Read the model definition and answer for the solid it produces. Units are mm, in the model's axes. Face numbers are marked on the shaded views. A direction names the side the tool comes from. Round coordinates to 2 decimals unless told otherwise and drop trailing zeros. Order: outer loops, then holes, each group sorted by start corner. A loop starts at its lowest first (then second) coordinate and runs counter-clockwise, first axis right, second up.
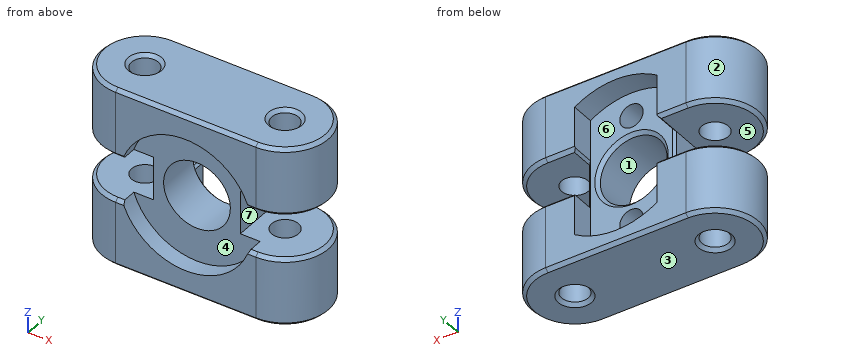
from build123d import *

# Parameters (mm, degrees)
SKETCH1_W           = 21
SKETCH1_H           = 27
BOSS_EXTRUDE1_DEPTH = 13
SKETCH8_R           = 6.5
BOSS_EXTRUDE2_DEPTH = 27
SKETCH2_R           = 5
CUT_EXTRUDE1_DEPTH  = 13
SKETCH3_W           = 21.50173114
SKETCH3_H           = 6.5
CUT_EXTRUDE2_DEPTH  = 13
SKETCH7_W           = 13
SKETCH7_H           = 6.5
CUT_EXTRUDE7_DEPTH  = 3.5
SKETCH4_R           = 2
CUT_EXTRUDE3_DEPTH  = 35
CUT_EXTRUDE4_DEPTH  = 3.5
SKETCH6_R           = 1.75
CUT_EXTRUDE5_DEPTH  = 6
CHAMFER1_SIZE       = 0.5
CHAMFER2_SIZE       = 0.35
CHAMFER3_SIZE       = 0.35
SKETCH9_R           = 10
CUT_EXTRUDE8_DEPTH  = 2.5


with BuildPart() as part:
    # Sketch1 → Boss-Extrude1 (new body)
    with BuildSketch(Plane(origin=(0, 0, 0), x_dir=(1, 0, 0), z_dir=(0, 1, 0))):
        Rectangle(SKETCH1_W, SKETCH1_H)
    extrude(amount=BOSS_EXTRUDE1_DEPTH)

    # Sketch8 → Boss-Extrude2 (add)
    with BuildSketch(Plane(origin=(0, 0, -13.5), x_dir=(-1, 0, 0), z_dir=(0, 0, -1))):
        with Locations((-10.5, 6.5)):
            Circle(SKETCH8_R)
        with Locations((10.5, 6.5)):
            Circle(SKETCH8_R)
    extrude(amount=-BOSS_EXTRUDE2_DEPTH)

    # Sketch2 → Cut-Extrude1 (cut)
    with BuildSketch(Plane(origin=(0, 13, 0), x_dir=(1, 0, 0), z_dir=(0, 1, 0))):
        with Locations(Location((0, 0, 0), (0, 0, 270))):
            Circle(SKETCH2_R)
    extrude(amount=-CUT_EXTRUDE1_DEPTH, mode=Mode.SUBTRACT)

    # Sketch3 → Cut-Extrude2 (cut)
    with BuildSketch(Plane(origin=(0, 13, 0), x_dir=(1, 0, 0), z_dir=(0, 1, 0))):
        with Locations((17.25086557, 0)):
            Rectangle(SKETCH3_W, SKETCH3_H)
        with Locations((-17.25086557, 0)):
            Rectangle(SKETCH3_W, SKETCH3_H)
    extrude(amount=-CUT_EXTRUDE2_DEPTH, mode=Mode.SUBTRACT)

    # Sketch7 → Cut-Extrude7 (cut)
    with BuildSketch(Plane(origin=(0, 13, 0), x_dir=(1, 0, 0), z_dir=(0, 1, 0))):
        Rectangle(SKETCH7_W, SKETCH7_H)
    extrude(amount=-CUT_EXTRUDE7_DEPTH, mode=Mode.SUBTRACT)

    # Sketch4 → Cut-Extrude3 (cut)
    with BuildSketch(Plane.XY.offset(13.5)):
        with Locations((-10.5, 6.5)):
            Circle(SKETCH4_R)
        with Locations((10.5, 6.5)):
            Circle(SKETCH4_R)
    extrude(amount=-CUT_EXTRUDE3_DEPTH, mode=Mode.SUBTRACT)

    # Sketch5 → Cut-Extrude4 (cut)
    with BuildSketch(Plane(origin=(0, 13, 0), x_dir=(1, 0, 0), z_dir=(0, 1, 0))):
        with BuildLine():
            Line((-6.15, 9.717381334), (-6.15, -9.717381334))
            ThreePointArc((-6.15, -9.717381334), (0, -11.5), (6.15, -9.717381334))
            Line((6.15, -9.717381334), (6.15, 9.717381334))
            ThreePointArc((6.15, 9.717381334), (0, 11.5), (-6.15, 9.717381334))
        make_face()
    extrude(amount=-CUT_EXTRUDE4_DEPTH, mode=Mode.SUBTRACT)

    # Sketch6 → Cut-Extrude5 (cut)
    with BuildSketch(Plane(origin=(0, 9.5, 0), x_dir=(1, 0, 0), z_dir=(0, 1, 0))):
        with Locations(Location((0, 8, 0), (0, 0, 270))):
            Circle(SKETCH6_R)
        with Locations(Location((0, -8, 0), (0, 0, 270))):
            Circle(SKETCH6_R)
    extrude(amount=-CUT_EXTRUDE5_DEPTH, mode=Mode.SUBTRACT)

    # Chamfer1
    chamfer1_edges = [part.edges().sort_by_distance(p)[0] for p in [
        (-12.5, 6.5, -13.5),
        (-12.5, 6.5, 13.5),
        (8.5, 6.5, -13.5),
        (8.5, 6.5, 13.5),
        (8.325, 13, 3.25),
        (-8.325, 13, -3.25),
        (17, 6.5, -13.5),
        (17, 6.5, 13.5),
        (0, 13, 13.5),
        (-17, 6.5, -13.5),
        (-17, 6.5, 13.5),
        (0, 0, -5),
        (-17, 6.5, -3.25),
        (-17, 6.5, 3.25),
        (17, 6.5, -3.25),
        (17, 6.5, 3.25),
        (8.5, 0, 3.25),
        (8.5, 0, -3.25),
        (8.325, 13, -3.25),
        (0, 0, 13.5),
        (-8.5, 0, 3.25),
        (-8.5, 0, -3.25),
        (0, 0, -13.5),
        (-8.325, 13, 3.25),
        (0, 9.5, -5),
        (0, 13, -13.5),
    ]]
    chamfer(chamfer1_edges, length=CHAMFER1_SIZE)

    # Chamfer2
    chamfer2_edges = [part.edges().sort_by_distance(p)[0] for p in [
        (6.15, 11, 3.25),
        (6.15, 11, -3.25),
        (-6.15, 11, -3.25),
        (-6.15, 11, 3.25),
    ]]
    chamfer(chamfer2_edges, length=CHAMFER2_SIZE)

    # Chamfer3
    chamfer3_edges = [part.edges().sort_by_distance(p)[0] for p in [
        (6.5, 9.5, 0),
        (-6.5, 9.5, 0),
        (-6.5, 0, 0),
        (6.5, 0, 0),
    ]]
    chamfer(chamfer3_edges, length=CHAMFER3_SIZE)

    # Sketch9 → Cut-Extrude8 (cut)
    with BuildSketch(Plane.XZ):
        Circle(SKETCH9_R)
    extrude(amount=-CUT_EXTRUDE8_DEPTH, mode=Mode.SUBTRACT)


solid = part.part
Q1. A cutting plane is placed at B-B, the plane x = 7. Give the vertices of the cut face in (y, z).
Outcome:
outline: (0, -13) - (0.5, -13.5) - (12.5, -13.5) - (13, -13) - (13, -3.75) - (12.5, -3.25) - (2.5, -3.25) - (2.5, -7.14) - (0, -7.14) - close; (0, 7.14) - (2.5, 7.14) - (2.5, 3.25) - (12.5, 3.25) - (13, 3.75) - (13, 13) - (12.5, 13.5) - (0.5, 13.5) - (0, 13) - close
Q2. A cutting plane is placed at A-A, the plane z = 8. Give the vertices of the cut face in (x, y).
Outcome:
outline: (-10.5, 0) - (-6, 0) - (-6, 2.5) - (6, 2.5) - (6, 0) - (10.5, 0) arc R6.5 ccw to (10.5, 13) - (6.15, 13) - (6.15, 9.5) - (1.75, 9.5) - (1.75, 3.5) - (-1.75, 3.5) - (-1.75, 9.5) - (-6.15, 9.5) - (-6.15, 13) - (-10.5, 13) arc R6.5 ccw to start; hole circle Ø4 at (-10.5, 6.5); hole circle Ø4 at (10.5, 6.5)
Q3. A cutting plane is placed at D-D, the plane z = -8.5. Give the vertices of the cut face in (x, y), plus the area to 3 significant figures.
Outcome:
outline: (-10.5, 0) - (-5.27, 0) - (-5.27, 2.5) - (5.27, 2.5) - (5.27, 0) - (10.5, 0) arc R6.5 ccw to (10.5, 13) - (6.15, 13) - (6.15, 9.5) - (1.68, 9.5) - (1.68, 3.5) - (-1.68, 3.5) - (-1.68, 9.5) - (-6.15, 9.5) - (-6.15, 13) - (-10.5, 13) arc R6.5 ccw to start; hole circle Ø4 at (-10.5, 6.5); hole circle Ø4 at (10.5, 6.5)
area: 291 mm2
Q4. Flat-ended cylindrical pins translate along their axes: pin 1 (4.5 mm diameter, centred on x = -10.5, y = 6.5, fed in from +Z); pin 2 (4 mm diameter, centred on x = -0.5, z = 7.5, fed in from +Y); pin 3 (1.5 mm diameter, centred on x = -11.5, z = -7, fed in from -Y). Find the tip coordinate at first contact, or state that the pin passes through.
Outcome:
pin 1: stops at z = 13.25
pin 2: stops at y = 9.5
pin 3: stops at y = 0
Q5. Straight lines are drawn through the part: probe 1 along Y at (x, z) = (10.5, 5.75); probe 2 along X at (y, z) = (6.75, -11.5); probe 3 along X at (y, z) = (5.75, 0). For each, find the intervals that lie inside material, in ascending order.
Outcome:
probe 1: y = 0 to 4.5, 8.5 to 13
probe 2: x = -17 to -12.48, -8.52 to 8.52, 12.48 to 17
probe 3: x = -6.5 to -5, 5 to 6.5
Q6. For a pull along Z with two mould halves and no side action, classify the marked faces 1, 2 and 3 as released by +Z, released by -Z, zero draft, split by the parting line, or undercut.
Outcome:
face 1: undercut
face 2: zero draft
face 3: released by -Z
Q7. For the marked faces 4, 5, 6 and 7, determine the directions among +Z, -Z, +X, -X, +Y, -Y from which every point of the face is accessible in a straight line to the end or side of a thin tool.
Outcome:
face 4: -Y
face 5: -X, +Y, -Y
face 6: +Y
face 7: +X, +Y, -Y
Q8. A cutting plane is placed at C-C, the plane y = 6.5. Give the number of separate pieces and of enclosed holes in the cut face, plus the area to 3 significant figures.
Outcome:
separate pieces: 5
enclosed holes: 3
area: 518 mm2
